```python
from build123d import *

# Parameters (mm, degrees)
SKETCH_1_W     = 81
SKETCH_1_H     = 2.5
CHAMFER_1_SIZE = 0.5


with BuildPart() as part:
    # Эскиз1 → Повернуть1 (revolve)
    with BuildSketch(Plane.XY):
        with Locations((40.5, 11.25)):
            Rectangle(SKETCH_1_W, SKETCH_1_H)
    revolve(axis=Axis((0, 0, 0), (1, 0, 0)))

    # Фаска1
    chamfer_1_edges = [part.edges().sort_by_distance(p)[0] for p in [
        (81, -12.5, 0),
        (81, -10, 0),
        (0, -10, 0),
        (0, -12.5, 0),
    ]]
    chamfer(chamfer_1_edges, length=CHAMFER_1_SIZE)


solid = part.part
```
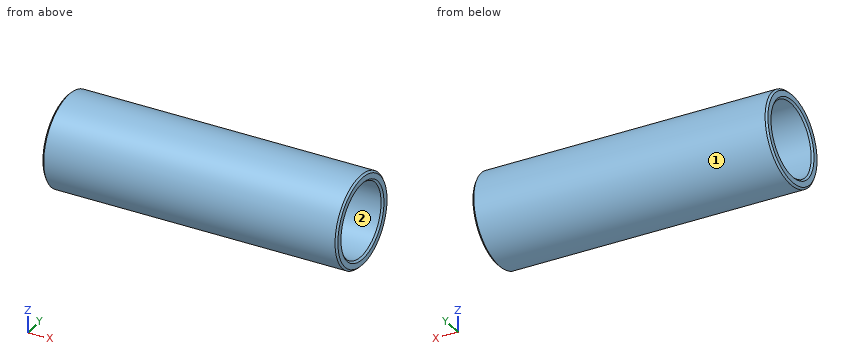
Model file for the job. Use its own axes, mm. Face numbers are marked on the shaded views. Coordinates: 2 decimals unless noted, no trailing zeros. Loops run counter-clockwise (first coordinate to the right, second up) from the corner with the lowest first, then second, coordinate; pieces in that order, holes last. Notation, with made-up numbers: (-22, 14) - (16, 14) arc R9 ccw to (16, 29) - close; hole circle Ø6 at (-32.75, 35.25). An arc over 180 degrees is marked (long way). Answer as a JSON object with one key per item and string values. Group by question number.
(1) Cut at A-A (z = 0). Give the cut face in (x, y), then the cut area to 3 significant figures.
(2) Cut at C-C (x = 50). Give the cut face in (y, z).
(3) Two-plate mould, pull along Y, no slides. Class the marked faces 1 and 2: released by +Y, released by -Y, zero draft, split by the parting line, or undercut.
(4) Probe line 1 along Y through (x, z) = (61, -0.25); line 2 along Y through (x, z) = (7.5, 4). List the from-to ranges inside material, lowest first.
(5) Flat gauge pins, fed straight in: pin 1 (5 mm diameter, centred on x = 31, z = -6, fed in from -Y); pin 2 (1 mm diameter, centred on x = 20, y = 4.5, fed in from +Z); pin 3 (1.5 mm diameter, centred on x = 39, z = -9.5, fed in from -Y). Where does each tip first touch, or does it go through?
Geometry says:
{
 "1": {"outline": "(0, -12) - (0.5, -12.5) - (80.5, -12.5) - (81, -12) - (81, -10.5) - (80.5, -10) - (0.5, -10) - (0, -10.5) - close; (0, 10.5) - (0.5, 10) - (80.5, 10) - (81, 10.5) - (81, 12) - (80.5, 12.5) - (0.5, 12.5) - (0, 12) - close", "area": "404 mm^2"},
 "2": {"outline": "circle Ø25 at (0, 0); hole circle Ø20 at (0, 0)"},
 "3": {"face 1": "split by the parting line", "face 2": "undercut"},
 "4": {"line 1": "y = -12.5 to -10, 10 to 12.5", "line 2": "y = -11.84 to -9.17, 9.17 to 11.84"},
 "5": {"pin 1": "stops at y = -12", "pin 2": "stops at z = 11.84", "pin 3": "stops at y = -8.93"}
}
